Part print with two shaded views. Sizes in mm from the minimum x, y, z corner. A direction names the side the tool comes from. Give positions to 0.01 mm unless a question says otherwise; leave off trailing zeros. Return JSON: item names as keys, results as strings. Group by question number.
Q1. Flat gauge pins, fed straight in: pin 1 Ø6 at (x, z) = (128, 53) entering from +Y; pin 2 Ø2 at (y, z) = (18, 67) entering from +X; pin 3 Ø11.5 at (x, z) = (79.27, 46.12) entering from +Y. Where does each tip first touch, or does it go through?
Q2. Pull direction Z, two halves, no side cores. Call the marked faces 1, 2 and 3: +Z half, -Z half, draft (parallel to the pull), parting line (faces both ways), or undercut.
Q3. Wall check: probe 1 along X at (y, z) = (6, 12); probe 2 along Y at (x, z) = (91, 15); probe 3 along X at (y, z) = (47, 41). Give the ranges that are in metal, low to high.
Q4. Tool access for the marked faces 4, 5 and 6: list every direction of +Z, -Z, +X, -X, +Y, -Y with a clear straight run to the whole face (end or side of a thin tool).
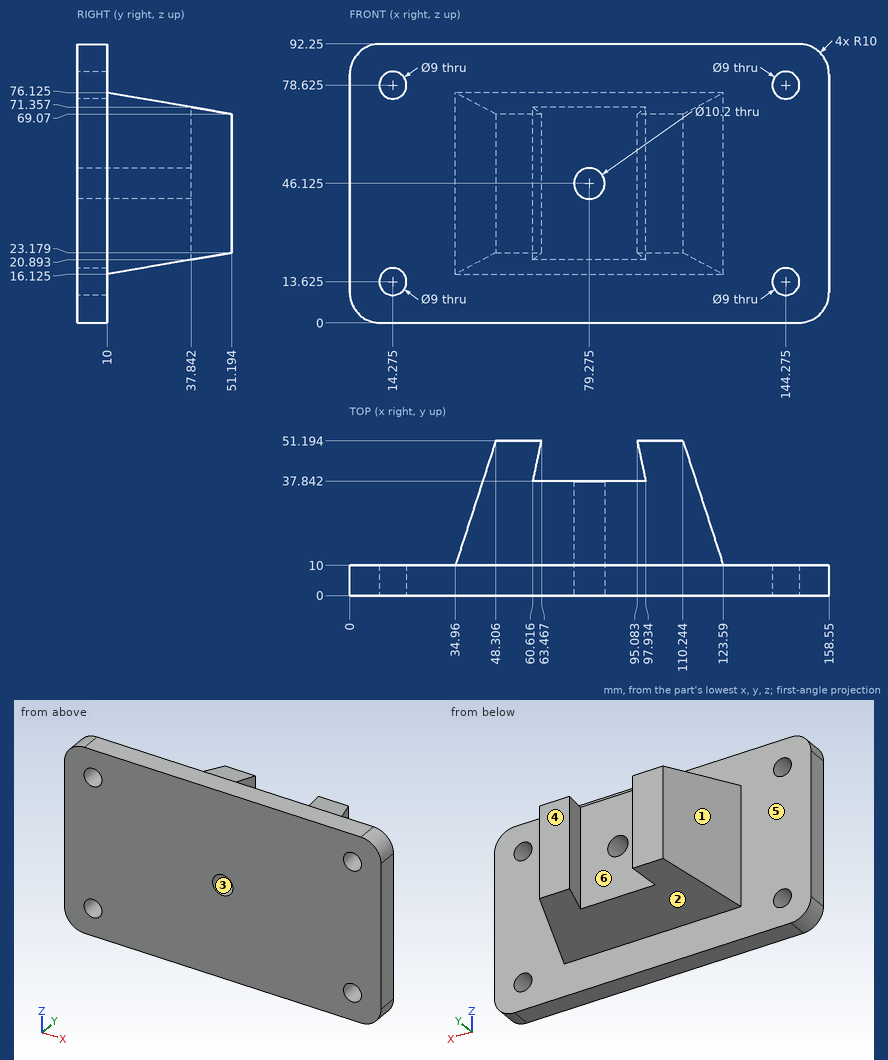
From the geometry:
{
 "1": {"pin 1": "stops at y = 10", "pin 2": "stops at x = 121.32", "pin 3": "stops at y = 37.84"},
 "2": {"face 1": "draft", "face 2": "-Z half", "face 3": "undercut"},
 "3": {"probe 1": "x = 0 to 10.08, 18.47 to 140.08, 148.47 to 158.55", "probe 2": "y = 0 to 10", "probe 3": "x = 46.95 to 62.57, 95.98 to 111.6"},
 "4": {"face 4": "+Z, -Z, +X, -X, +Y", "face 5": "+Y", "face 6": "+Z, -Z"}
}
